Could you check a few things on this model? Use its own coordinates, in mm. A direction names the side the tool comes from. Give positions to 0.01 mm unless a question says otherwise; leave off trailing zeros. Loops run counter-clockwise (first coordinate to the right, second up) from the corner with the lowest first, then second, coordinate; pieces in that order, holes last. Notation, with made-up numbers: M -30,30.5 L 16,30.5 A29 cw 16,62.5 Z; hole C 45,-17.5 d9. An arc over 180 degrees is marked long. Answer in a Markdown table with one row per item. Add a question column.
1. If we section it at A-A on y = 22: List the corners of the cut face in (x, z) for me.
2. I'm going to push flat-ended pins straight in: pin 1 Ø6 at (y, z) = (-1.5, 9.5) entering from -X; pin 2 Ø5 at (x, z) = (-135, 17) entering from -Y; pin 3 Ø7.5 at (x, z) = (-131, 6) entering from +Y; pin 4 Ø1 at (x, y) = (-128.5, -54.5) entering from +Z. Where does each tip first touch, or does it pass through?
3. If we section it at B-B on x = -125: Count the separate pieces of the cut face and the enclosed holes in it, then the cut area to 3 significant figures.
4. Thinking about a two-plate mould opening in Z: for faces 5 (the flat face through (-126.2, -9.2, 5)), 6 (the flat face through (-135, 24, 15)), 7 (the flat face through (-127, 22, -5)), which applies, released by +Z, released by -Z, zero draft, split by the parting line, or undercut?
5. If we section it at C-C on y = -8: List the corners of the cut face in (x, z) for me.
6. I need wall thicknesses on line 1 along Y through (x, z) = (-130.25, 17.5); line 2 along Y through (x, z) = (-135, 8); line 3 along Y through (x, z) = (-125.25, 5.5). Which ranges of each line are inside material? Lowest first, please. Write a range as from..to.
7. Which directions (+Z, -Z, +X, -X, +Y, -Y) give clear straight access to the entire face, cutting with the end or side of a thin tool? Please do faces 1 (the flat face through (-135, 15, 8)), 2 (the flat face through (-130, -41, 2)), 3 (the flat face through (-127, -8, 10)), 4 (the flat face through (-135, 19, 15)).
```python
from build123d import *

# Parameters (mm, degrees)
PAD008_DEPTH         = 5
PAD009_DEPTH         = 10
PAD009_DEPTH_BACK    = 5
SKETCH045_W          = 10
SKETCH045_H          = 5
POCKET004_DEPTH      = 11
SKETCH044_R          = 1.5
POCKET005_DEPTH      = 10
PAD010_DEPTH         = 10
PAD010_DEPTH_BACK    = 5
SKETCH042_W          = 10
SKETCH042_H          = 5
POCKET006_DEPTH      = 10
SKETCH041_R          = 1.5
POCKET007_DEPTH      = 15
FILLET_R             = 2
FILLET001_R          = 6
FILLET002_R          = 2
SKETCH039_W          = 10
SKETCH039_H          = 2
SKETCH039_H_2        = 4
PAD021_DEPTH         = 10
PAD022_DEPTH         = 20
POCKET018_DEPTH      = 8
PAD025_DEPTH         = 6
FILLET003_R          = 3
SKETCH040_R          = 1.5
POCKET023_DEPTH      = 15
POCKET023_DEPTH_BACK = 6


with BuildPart() as part:
    # Sketch047 → Pad008 (new body)
    with BuildSketch(Plane.XY):
        Polygon((0, 0), (5, 0), (5, -140), (-5, -140), (-5, 0), align=None)
    extrude(amount=PAD008_DEPTH)

    # Sketch046 → Pad009 (join, two sides)
    with BuildSketch(Plane.XY) as pad009_sk:
        Polygon((0, 0), (-5, 0), (-5, -10), (15, -10), (15, 0), align=None)
    extrude(amount=PAD009_DEPTH)
    extrude(pad009_sk.sketch, amount=-PAD009_DEPTH_BACK)

    # Sketch045 → Pocket004 (cut)
    with BuildSketch(Plane.YZ.offset(5)):
        with Locations((-5, 2.5)):
            Rectangle(SKETCH045_W, SKETCH045_H)
    extrude(amount=POCKET004_DEPTH, mode=Mode.SUBTRACT)

    # Sketch044 → Pocket005 (cut, symmetric)
    with BuildSketch(Plane(origin=(10, -5, 0), x_dir=(1, 0, 0), z_dir=(0, 0, 1))):
        Circle(SKETCH044_R)
    extrude(amount=POCKET005_DEPTH, both=True, mode=Mode.SUBTRACT)

    # Sketch043 → Pad010 (join, two sides)
    with BuildSketch(Plane.XY) as pad010_sk:
        Polygon((0, -30), (-5, -30), (-5, -40), (15, -40), (15, -30), align=None)
    extrude(amount=PAD010_DEPTH)
    extrude(pad010_sk.sketch, amount=-PAD010_DEPTH_BACK)

    # Sketch042 → Pocket006 (cut)
    with BuildSketch(Plane.YZ.offset(5)):
        with Locations((-35, 2.5)):
            Rectangle(SKETCH042_W, SKETCH042_H)
    extrude(amount=POCKET006_DEPTH, mode=Mode.SUBTRACT)

    # Sketch041 → Pocket007 (cut)
    with BuildSketch(Plane(origin=(10, -35, 10), x_dir=(1, 0, 0), z_dir=(0, 0, 1))):
        Circle(SKETCH041_R)
    extrude(amount=-POCKET007_DEPTH, mode=Mode.SUBTRACT)

    # Fillet
    fillet_edges = [part.edges().sort_by_distance(p)[0] for p in [
        (-5, -20, 5),
        (-5, -90, 5),
        (-5, -90, 0),
        (-5, -20, 0),
    ]]
    fillet(fillet_edges, radius=FILLET_R)

    # Fillet001
    fillet001_edges = [part.edges().sort_by_distance(p)[0] for p in [
        (-5, -35, -5),
        (-5, -35, 10),
        (-5, -5, -5),
    ]]
    fillet(fillet001_edges, radius=FILLET001_R)

    # Fillet002
    fillet002_edges = [part.edges().sort_by_distance(p)[0] for p in [
        (5, -140, 2.5),
        (1, -140, 5),
        (-4.414214, -140, 4.414214),
        (-4.414214, -140, 0.585786),
        (1, -140, 0),
        (-5, -140, 2.5),
    ]]
    fillet(fillet002_edges, radius=FILLET002_R)

    # Sketch039 → Pad021 (join)
    with BuildSketch(Plane(origin=(-5, 0, 10), x_dir=(1, 0, 0), z_dir=(0, 0, 1))):
        with Locations((5, -1)):
            Rectangle(SKETCH039_W, SKETCH039_H)
        with Locations((5, -5)):
            Rectangle(SKETCH039_W, SKETCH039_H_2)
        with Locations((5, -9)):
            Rectangle(SKETCH039_W, SKETCH039_H)
    extrude(amount=PAD021_DEPTH)

    # Sketch048 → Pad022 (join)
    with BuildSketch(Plane.XY):
        Polygon((0, 0), (-3, 0), (-3, 3), (3, 3), (3, 0), align=None)
    extrude(amount=PAD022_DEPTH)

    # Sketch049 → Pocket018 (cut)
    with BuildSketch(Plane.YZ.offset(-3)):
        Polygon((0, 0), (3, 0), (3, 4), align=None)
        Polygon((3, 20), (1, 20), (1, 15), (3, 12), align=None)
        Polygon((0, 20), (0.2, 20), (0.2, 14.2), (2.1, 11.35), (2.1, 4.8), (0, 2), (0, 14.5), align=None)
    extrude(amount=POCKET018_DEPTH, mode=Mode.SUBTRACT)

    # Sketch054 → Pad025 (join)
    with BuildSketch(Plane(origin=(-3, -12, 5), x_dir=(0, 1, 0), z_dir=(1, 0, 0))):
        Polygon((0, 0), (0, 6), (1.6, 9), (1.6, 15), (0.6, 15), (0.6, 9), (-1, 6), (-1, 0), align=None)
    extrude(amount=PAD025_DEPTH)

    # Fillet003
    fillet003_edges = [part.edges().sort_by_distance(p)[0] for p in [
        (0, -12, 11),
        (0, -10.4, 14),
        (0, -13, 11),
        (0, -11.4, 14),
        (0, 2.1, 11.35),
        (0, 3, 4),
        (0, 3, 12),
        (0, 1, 15),
        (0, 0.2, 14.2),
        (0, 2.1, 4.8),
    ]]
    fillet(fillet003_edges, radius=FILLET003_R)

    # Sketch040 → Pocket023 (cut, two sides)
    with BuildSketch(Plane(origin=(0, -10, 17), x_dir=(1, 0, 0), z_dir=(0, -1, 0))) as pocket023_sk:
        Circle(SKETCH040_R)
    extrude(amount=-POCKET023_DEPTH, mode=Mode.SUBTRACT)
    extrude(pocket023_sk.sketch, amount=POCKET023_DEPTH_BACK, mode=Mode.SUBTRACT)


with BuildPart() as part_1:
    # Body007 placement: moved
    add(part.part.moved(Location((-135, 27, 0))))


solid = part_1.part
```
Results:
| question | item | result |
|---|---|---|
| 1 | outline | M -140,1 A6 ccw -134,-5 L -126.5,-5 L -126.5,0 L -130,0 L -130,5 L -126.5,5 L -126.5,10 L -130,10 L -130,20 L -140,20 Z; M -123.5,-5 L -120,-5 L -120,0 L -123.5,0 Z; M -123.5,5 L -120,5 L -120,10 L -123.5,10 Z; hole C -135,17 d3 |
| 2 | pin 1 | x = -139.25 |
| 2 | pin 2 | y = 15.59 |
| 2 | pin 3 | y = 30 |
| 2 | pin 4 | through |
| 3 | separate pieces | 8 |
| 3 | enclosed holes | 0 |
| 3 | area | 140 mm2 |
| 4 | face 5 | undercut |
| 4 | face 6 | zero draft |
| 4 | face 7 | released by -Z |
| 5 | outline | M -140,1 A6 ccw -134,-5 L -126.5,-5 L -126.5,0 L -130,0 L -130,5 L -126.5,5 L -126.5,10 L -134,10 A6 ccw -140,4 Z; M -123.5,-5 L -120,-5 L -120,0 L -123.5,0 Z; M -123.5,5 L -120,5 L -120,10 L -123.5,10 Z |
| 6 | line 1 | 17..19, 20..24, 25..27 |
| 6 | line 2 | -13..-3, 14..15, 17..27, 29.1..30 |
| 6 | line 3 | -13..-9.48, -6.52..-3, 17..20.52, 23.48..27 |
| 7 | face 1 | +X, -X |
| 7 | face 2 | +X, +Y, -Y |
| 7 | face 3 | +Z, +X, -X, -Y |
| 7 | face 4 | +Z, +X, -X |
